from build123d import *

# Parameters (mm, degrees)
F1_DEPTH = 25.4
F3_DEPTH = 25.401


with BuildPart() as f1:
    # F0 (on Front) → F1 (new body)
    with BuildSketch(Plane.XZ):
        Polygon((-28.907506, 44.009075), (-44.663455, 44.009075), (-44.663455, -35.910148), (29.924411, -35.910148), (29.924411, -21.110609), align=None)
    extrude(amount=F1_DEPTH)

    # F2 (on face) → F3 (cut, through all)
    with BuildSketch(Plane.XZ.offset(25.4)):
        Polygon((-21.82091, 18.790228), (-34.549773, 18.790228), (-34.549773, -22.427047), (8.182841, -22.427047), (8.182841, -16.971819), align=None)
    extrude(amount=-F3_DEPTH, mode=Mode.SUBTRACT)


solid = f1.part
Work out the finished part from the listing and answer in its coordinate system (mm). A direction names the side the tool comes from. Give positions to 0.01 mm unless a question says otherwise; leave off trailing zeros. Order: outer loops, then holes, each group sorted by start corner. A loop starts at its lowest first (then second) coordinate and runs counter-clockwise, first axis right, second up. Notation, with made-up numbers: (84, -12.5) -> (135, -12.5) arc R29 cw to (135, 17.5) -> close; hole circle Ø1 at (-21, 26.5). An arc over 180 degrees is marked (long way). Answer as a JSON object with one key per item and string values. Group by question number.
1. Section A-A on x = -15 is taken. Determine the outline of the cut face in (y, z), plus the area to 3 significant figures.
2. Section B-B on z = -20 is taken. Determine the outline of the cut face in (x, y), plus the area to 3 significant figures.
3. A tool of negligible diameter and unlimited length cuts with its end or side. For faces 5 (the flat face through (-8, -13, -35.91)), 6 (the flat face through (8.183, -13, -20)), from which of +Z, -Z, +X, -X, +Y, -Y can it reach the whole face along a straight path? Write none if from no direction.
4. Section C-C on y = -10.25 is taken. Determine the outline of the cut face in (x, z), plus the area to 3 significant figures.
5. Section D-D on z = 37 is taken. Determine the outline of the cut face in (x, y).
6. Consider line 1 along X through (y, z) = (-10.75, -14); line 2 along X through (y, z) = (-18, 0.5); line 3 along Z through (x, y) = (-25, -4.5). Determine where each line is inside the solid, lowest interval first. Write a range as [from, to].
7. Flat-ended cylindrical pins translate along their axes: pin 1 Ø1.5 at (x, z) = (18, -27.5) entering from +Y; pin 2 Ø7.5 at (x, y) = (-6, -16.5) entering from +Z; pin 3 Ø3 at (y, z) = (-23, 26.5) entering from +X. Find the tip coordinate at first contact, or state that the pin passes through.
8. The mould has two halves that part along Z. Classify faces 1 (the flat face through (29.924, -13, -29)), 2 (the flat face through (-13, -13, -22.427)), 3 (the flat face through (-28, -13, 18.79)), 4 (the flat face through (0.92, -12.522, 10.993)): released by +Z, released by -Z, zero draft, split by the parting line, or undercut.
Result sheet:
{
 "1": {"outline": "(-25.4, -35.91) -> (0, -35.91) -> (0, -22.43) -> (-25.4, -22.43) -> close; (-25.4, 10.66) -> (0, 10.66) -> (0, 28.62) -> (-25.4, 28.62) -> close", "area": "799 mm^2"},
 "2": {"outline": "(-44.66, -25.4) -> (-34.55, -25.4) -> (-34.55, 0) -> (-44.66, 0) -> close; (8.18, -25.4) -> (28.92, -25.4) -> (28.92, 0) -> (8.18, 0) -> close", "area": "784 mm^2"},
 "3": {"face 5": "-Z, +X, -X, +Y, -Y", "face 6": "+Y, -Y"},
 "4": {"outline": "(-44.66, -35.91) -> (29.92, -35.91) -> (29.92, -21.11) -> (-28.91, 44.01) -> (-44.66, 44.01) -> close; hole (-34.55, -22.43) -> (8.18, -22.43) -> (8.18, -16.97) -> (-21.82, 18.79) -> (-34.55, 18.79) -> close", "area": "2,820 mm^2"},
 "5": {"outline": "(-44.66, -25.4) -> (-22.58, -25.4) -> (-22.58, 0) -> (-44.66, 0) -> close"},
 "6": {"line 1": "x = [-44.66, -34.55], [5.69, 23.5]", "line 2": "x = [-44.66, -34.55], [-6.48, 10.4]", "line 3": "z = [-35.91, -22.43], [18.79, 39.68]"},
 "7": {"pin 1": "stops at y = 0", "pin 2": "stops at z = 22.8", "pin 3": "stops at x = -11.73"},
 "8": {"face 1": "zero draft", "face 2": "undercut", "face 3": "undercut", "face 4": "released by +Z"}
}
